Design review of the part built by this model. Coordinates are the model's own, in mm. A direction names the side the tool comes from. Coordinates: 2 decimals unless noted, no trailing zeros. Write each loop counter-clockwise with the first axis right and the second up, starting at its lowest first coordinate (ties: lowest second). Pieces come first, ordered by that corner, then holes.
Q1. Take a section at A-A, the plane y = 5. Write out the cut boundary in (x, z), plus the area to 3 significant figures.
Q2. The part is to be moulded in two halves that separate along Y. For faces 3 (the flat face through (4, 12, 1)), 4 (the flat face through (12, -5, 1)), 5 (the flat face through (30, 12, 1)), say which applies: released by +Y, released by -Y, zero draft, split by the parting line, or undercut.
Q3. Take a section at C-C, the plane x = 2. Write out the cut boundary in (y, z), plus the area to 3 significant figures.
Q4. Take a section at B-B, the plane x = 6. Write out the cut boundary in (y, z).
Q5. For pin 1 Ø3.5 at (x, y) = (27.5, -2.5) entering from +Z, flat-tipped, find the tip position at first contact; note if it passes through.
Q6. For L1, parallel to Y at x = 23, z = 1.35; L2, parallel to Y at x = -2.5, z = 1.8; L3, parallel to X at y = 0.5, z = 1.6, list the stretches that pass through material, from the lowest coordinate up.
Q7. Take a section at D-D, the plane y = -2.5. Write out the cut boundary in (x, z), plus the area to 3 significant figures.
Q8. For faces 1 (the flat face through (21, 12, 1)), 2 (the flat face through (-5, 12, 1)), list the 3-axis set-ups (+Z, -Z, +X, -X, +Y, -Y) from which the entire face can be reached by the end or side of a thin tool; tool diameter is ignored.
from build123d import *

# Parameters (mm, degrees)
SKETCH1_W           = 35
SKETCH1_H           = 35
SKETCH1_W_2         = 17
SKETCH1_H_2         = 25
SKETCH1_R           = 1.1
SKETCH1_R_2         = 1.624281561
BOSS_EXTRUDE1_DEPTH = 3


with BuildPart() as part:
    # Sketch1 → Boss-Extrude1 (new body)
    with BuildSketch(Plane.XY):
        with Locations((12.5, 12.5)):
            Rectangle(SKETCH1_W, SKETCH1_H)
        with Locations((12.5, 12.5)):
            Rectangle(SKETCH1_W_2, SKETCH1_H_2, mode=Mode.SUBTRACT)
        with Locations((2, 2)):
            Circle(SKETCH1_R, mode=Mode.SUBTRACT)
        with Locations((2, 14.5)):
            Circle(SKETCH1_R, mode=Mode.SUBTRACT)
        with Locations((-2.5, -2.5)):
            Circle(SKETCH1_R_2, mode=Mode.SUBTRACT)
        with Locations((27.5, -2.5)):
            Circle(SKETCH1_R_2, mode=Mode.SUBTRACT)
        with Locations((-2.5, 27.5)):
            Circle(SKETCH1_R_2, mode=Mode.SUBTRACT)
        with Locations((27.5, 27.5)):
            Circle(SKETCH1_R_2, mode=Mode.SUBTRACT)
        with Locations((23, 14.5)):
            Circle(SKETCH1_R, mode=Mode.SUBTRACT)
        with Locations((23, 2)):
            Circle(SKETCH1_R, mode=Mode.SUBTRACT)
    extrude(amount=BOSS_EXTRUDE1_DEPTH)


solid = part.part
Responses:
1. outline: (-5, 0) - (4, 0) - (4, 3) - (-5, 3) - close; (21, 0) - (30, 0) - (30, 3) - (21, 3) - close
1. area: 54.0 mm2
2. face 3: undercut
2. face 4: released by -Y
2. face 5: zero draft
3. outline: (-5, 0) - (0.9, 0) - (0.9, 3) - (-5, 3) - close; (3.1, 0) - (13.4, 0) - (13.4, 3) - (3.1, 3) - close; (15.6, 0) - (30, 0) - (30, 3) - (15.6, 3) - close
3. area: 91.8 mm2
4. outline: (-5, 0) - (0, 0) - (0, 3) - (-5, 3) - close; (25, 0) - (30, 0) - (30, 3) - (25, 3) - close
5. pin 1: stops at z = 3
6. L1: y = -5 to 0.9, 3.1 to 13.4, 15.6 to 30
6. L2: y = -5 to -4.12, -0.88 to 25.88, 29.12 to 30
6. L3: x = -5 to 4, 21 to 30
7. outline: (-5, 0) - (-4.12, 0) - (-4.12, 3) - (-5, 3) - close; (-0.88, 0) - (25.88, 0) - (25.88, 3) - (-0.88, 3) - close; (29.12, 0) - (30, 0) - (30, 3) - (29.12, 3) - close
7. area: 85.5 mm2
8. face 1: +Z, -Z
8. face 2: +Z, -Z, -X, +Y, -Y
